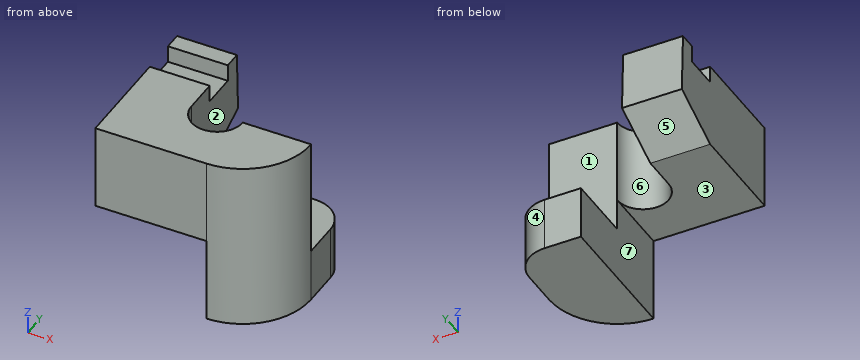
```python
from build123d import *

# Parameters (mm, degrees)
PAD_DEPTH    = 40
PAD003_DEPTH = 28
PAD004_DEPTH = 40
POCKET_DEPTH = 40
PAD005_DEPTH = 25


with BuildPart() as part:
    # Sketch → Pad (new body)
    with BuildSketch(Plane.XY):
        with BuildLine():
            Line((28, 32), (28, 48))
            Line((28, 48), (0, 48))
            Line((0, 48), (0, 0))
            Line((0, 0), (52, 0))
            ThreePointArc((52, 0), (74.627417, 9.372583), (84, 32))
            Line((84, 32), (52, 32))
            ThreePointArc((28, 32), (40, 19.999968), (52, 32))
        make_face()
    extrude(amount=PAD_DEPTH)

    # Sketch003 → Pad003 (join)
    with BuildSketch(Plane(origin=(0, 0, 0), x_dir=(0, -1, 0), z_dir=(-1, 0, 0))):
        Polygon((-48, 0), (-73, 12), (-72, 40), (-64, 40), (-64, 32), (-48, 32), align=None)
    extrude(amount=-PAD003_DEPTH)

    # Pad003 Face5 → Pad004 (add)
    with BuildSketch(Plane(origin=(34.657962, 19.802966, 0), x_dir=(0, -1, 0), z_dir=(0, 0, -1))):
        with BuildLine():
            Line((-28.197034, 6.657962), (-12.197034, 6.657962))
            ThreePointArc((-12.197034, 6.657962), (-0.197002, -5.342038), (-12.197034, -17.342038))
            Line((-12.197034, -17.342038), (-12.197034, -49.342038))
            ThreePointArc((-12.197034, -49.342038), (10.430383, -39.969455), (19.802966, -17.342038))
            Line((19.802966, -17.342038), (19.802966, 34.657962))
            Line((19.802966, 34.657962), (-28.197034, 34.657962))
            Line((-28.197034, 34.657962), (-28.197034, 6.657962))
        make_face()
    extrude(amount=PAD004_DEPTH)

    # Sketch004 (on Face16 of Pad004) → Pocket (cut)
    with BuildSketch(Plane(origin=(0, 0, -40), x_dir=(1, 0, 0), z_dir=(0, 0, -1))):
        with BuildLine():
            Line((52, 0), (0, 0))
            Line((0, 0), (0, -48))
            Line((0, -48), (28, -48))
            Line((28, -48), (28, -31.999968))
            ThreePointArc((52, -32), (40.000016, -19.999968), (28, -31.999968))
            Line((52, -32), (52, 0))
        make_face()
    extrude(amount=-POCKET_DEPTH, mode=Mode.SUBTRACT)

    # Sketch005 (on Face20 of Pocket) → Pad005 (join)
    with BuildSketch(Plane(origin=(0, 0, -40), x_dir=(1, 0, 0), z_dir=(0, 0, -1))):
        with BuildLine():
            Line((52, -32), (84, -32))
            Line((84, -32), (84, -49))
            ThreePointArc((69, -64), (79.606602, -59.606602), (84, -49))
            Line((69, -64), (52, -64))
            Line((52, -64), (52, -32))
        make_face()
    extrude(amount=-PAD005_DEPTH)


solid = part.part
```
Here's how the part is built. I have some questions about the finished solid (model axes, mm). Face numbers are marked on the shaded views. A direction names the side the tool comes from. Give positions to 0.01 mm unless a question says otherwise; leave off trailing zeros. Write each loop counter-clockwise with the first axis right and the second up, starting at its lowest first coordinate (ties: lowest second). Pieces come first, ordered by that corner, then holes. Notation, with made-up numbers: (65.25, 78.5) -> (87.25, 78.5) arc R8 ccw to (87.25, 92.5) -> close; hole circle Ø3 at (-34, 53). An arc over 180 degrees is marked (long way). Use one line per item in the form item = value.
1) I'm going to push flat-ended pins straight in: pin 1 (5 mm diameter, centred on x = 72, z = 2.5, fed in from +Y); pin 2 (9 mm diameter, centred on x = 18.5, z = 34.5, fed in from +Y); pin 3 (10 mm diameter, centred on x = 18.5, y = 35.5, fed in from -Z). Where does each tip first touch, or does it pass through?
Verdict:
pin_1 = 32
pin_2 = 72.36
pin_3 = 0
2) If I drill on L1, parallel to X at y = 54, z = 20; L2, parallel to X at y = 46.5, z = -16; L3, parallel to Z at x = 17.5, y = 24, over which ranges is the centre line in solid material (lowest first)? Write a range as [from, to].
Verdict:
L1 = [0, 28]
L2 = [52, 84]
L3 = [0, 40]
3) Suppose I cut it at A-A (y = 40). Please give me the cut outline in (x, z), and give its area (3 significant figures).
Verdict:
outline = (0, 0) -> (28, 0) -> (28, 40) -> (0, 40) -> close; (52, -40) -> (84, -40) -> (84, -15) -> (52, -15) -> close
area = 1,920 mm2
4) Suppose I cut it at B-B (z = -35). Please give me the cut outline in (x, y).
Verdict:
outline = (52, 0) arc R32 ccw to (84, 32) -> (84, 49) arc R15 ccw to (69, 64) -> (52, 64) -> close
5) We'd pull the mould along X, two halves only. Please class the marked faces 4, 5, 6 and 7: +X half, -X half, draft (parallel to the pull), parting line (faces both ways), or undercut.
Verdict:
face_4 = +X half
face_5 = draft
face_6 = undercut
face_7 = -X half
6) On a 3-axis mill with a long thin cutter (end or side, diameter ignored), from which of +Z, -Z, +X, -X, +Y, -Y can I reach the whole of each face in a straight line? I mean the marked faces 1, 2 and 3. Say none if no direction works.
Verdict:
face_1 = +Z, +X, +Y
face_2 = +Z, -Z, +X, +Y
face_3 = -Z, -X, +Y, -Y
7) Suppose I cut it at D-D (z = 33.5). Please give me the cut outline in (x, y).
Verdict:
outline = (0, 0) -> (52, 0) arc R32 ccw to (84, 32) -> (52, 32) arc R12 cw to (28, 32) -> (28, 48) -> (0, 48) -> close; (0, 64) -> (28, 64) -> (28, 72.23) -> (0, 72.23) -> close
8) Suppose I cut it at C-C (x = 23). Please give me the cut outline in (y, z), and give its area (3 significant figures).
Verdict:
outline = (0, 0) -> (48, 0) -> (73, 12) -> (72, 40) -> (64, 40) -> (64, 32) -> (48, 32) -> (48, 40) -> (0, 40) -> close
area = 2,630 mm2
